Design review of the part shown in the three views and the two pictorial views. Dimensions are in mm from the part's minimum x, y and z. Give positions to 0.01 mm unless a question says otherwise; leave off trailing zeros. Order: outer loops, then holes, each group sorted by start corner. A loop starts at its lowest first (then second) coordinate and runs counter-clockwise, first axis right, second up.
Item 1: Consider section C-C (y = 31). Give the boundary of the cut face in (x, z), plus the area to 3 significant figures.
Item 2: For probe 1 along Y at (x, z) = (20.5, 2.5); probe 2 along X at (y, z) = (58, 4.5), list the stretches that pass through material, from the lowest coordinate up.
Item 3: Consider section A-A (x = 179). Give the boundary of the cut face in (y, z).
Item 4: Consider section B-B (z = 2). Give the number of separate pieces and of enclosed holes in the cut face, plus the area to 3 significant figures.
Item 5: For P1, Ø3, axis at x = 142.5, y = 83, coming from the -Z side; P2, Ø1.9, axis at y = 58, z = 4, coming from the +X side, all flat-tipped, find the tip position at first contact; note any pin that passes through.
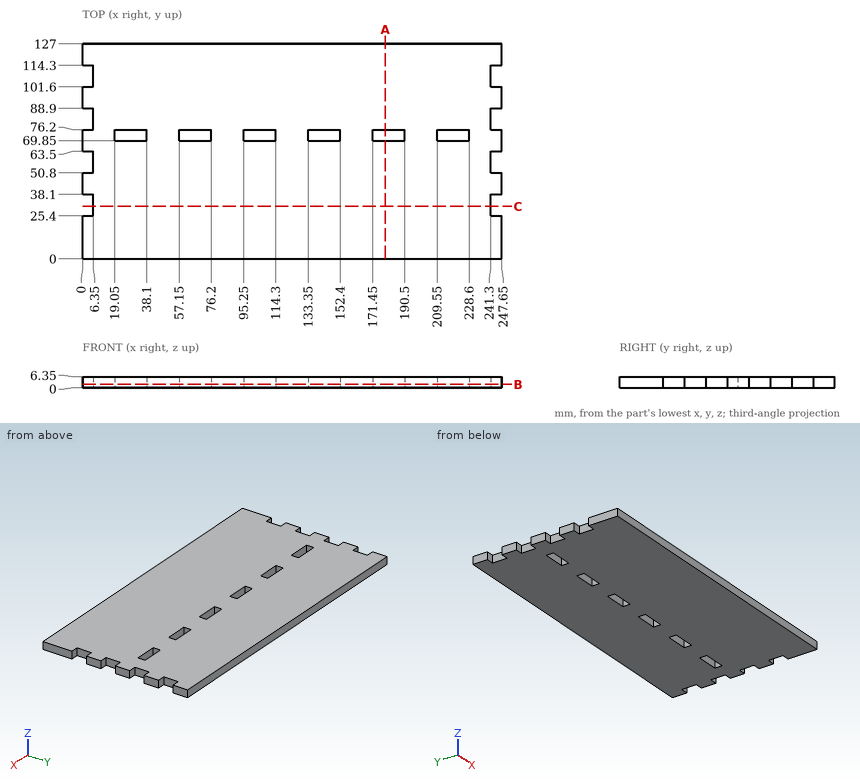
Resolved:
1. outline: (6.35, 0) - (241.3, 0) - (241.3, 6.35) - (6.35, 6.35) - close
1. area: 1,490 mm2
2. probe 1: y = 0 to 69.85, 76.2 to 127
2. probe 2: x = 6.35 to 241.3
3. outline: (0, 0) - (69.85, 0) - (69.85, 6.35) - (0, 6.35) - close; (76.2, 0) - (127, 0) - (127, 6.35) - (76.2, 6.35) - close
4. separate pieces: 1
4. enclosed holes: 6
4. area: 30,100 mm2
5. P1: stops at z = 0
5. P2: stops at x = 241.3
